Check sheet for the modelled part. Datum: model origin and axes. Units: mm. A direction names the side the tool comes from. Coordinates: 2 decimals unless noted, no trailing zeros. Order: outer loops, then holes, each group sorted by start corner. A loop starts at its lowest first (then second) coordinate and runs counter-clockwise, first axis right, second up.
1. Thickness scan on line 1 (Z direction, x = 1, y = -2); line 2 (X direction, y = 0.25, z = 2.75); line 3 (Y direction, x = -1, z = -5.5). Record the ranges inside material, lowest first.
2. Set-up check for faces 1 (the flat face through (1.3, -1.3, 6)), 2 (the flat face through (0, 0, 8)): record each of +Z, -Z, +X, -X, +Y, -Y from which the full face is reachable in a straight line by a thin tool's end or side.
3. Cross-section at A-A (z = -3.5). Enter the section's corners in (x, y).
4. Gauge pin test, flat ends, axial feed: pin 1 Ø3 at (x, y) = (-1, 2) entering from -Z; pin 2 Ø1 at (y, z) = (0, -11.5) entering from -X; pin 3 Ø1.5 at (x, z) = (2, -1) entering from +Y; pin 4 Ø1.5 at (x, z) = (1, -3) entering from -Y. Record the tip position at first contact, or that the pin passes through.
Autodesk Inventor part; units mm, degrees
ref_plane "YZ Plane" through (0, 0, 0) normal (1, 0, 0) x (0, 1, 0)
ref_plane "XZ Plane" through (0, 0, 0) normal (0, 1, 0) x (-1, 0, 0)
ref_plane "XY Plane" through (0, 0, 0) normal (0, 0, 1) x (1, 0, 0)
sketch "スケッチ1" plane through (0, 0, 0) normal (0, 0, 1) x (1, 0, 0)
  circle A0 centre (0, 0) radius 1.5
  dimension "d0" = 3
extrude "押し出し1" add sketch "スケッチ1" along normal blind 6
sketch "スケッチ2" plane through (0, 0, 6) normal (0, 0, 1) x (1, 0, 0)
  circle A0 centre (0, 0) radius 1.5
  circle A1 centre (0, 0) radius 3
  dimension "d3" = 6
extrude "押し出し2" add sketch "スケッチ2" along normal blind 2 contours A0 | A1
fillet "フィレット1" radius 2 1 edges at (-3, 0, 8)
thread "ねじ1"
sketch "スケッチ3" plane through (0, 0, 0) normal (0, 0, -1) x (-1, 0, 0)
  circle A0 centre (0, 0) radius 1.5
extrude "押し出し3" add sketch "スケッチ3" along normal blind 9
sketch "スケッチ4" plane through (0, 0, -9) normal (0, 0, -1) x (-1, 0, 0)
  circle A0 centre (0, 0) radius 1.5
extrude "押し出し4" add sketch "スケッチ4" along normal blind 10
properties part number "SB　25mmなべネジ" material "Steel, Mild"
Data:
1. line 1: z = 6 to 7.57
1. line 2: x = -1.48 to 1.48
1. line 3: y = -1.12 to 1.12
2. face 1: -Z
2. face 2: +Z, +X, -X, +Y, -Y
3. outline: circle Ø3 at (0, 0)
4. pin 1: stops at z = -19
4. pin 2: stops at x = -1.5
4. pin 3: stops at y = 0.83
4. pin 4: stops at y = -1.48
